Geometry check sheet. Reference: the model listing, model coordinates, mm. A direction names the side the tool comes from. Coordinates: 2 decimals unless noted, no trailing zeros. Order: outer loops, then holes, each group sorted by start corner. A loop starts at its lowest first (then second) coordinate and runs counter-clockwise, first axis right, second up. Notation, with made-up numbers: M -38.5,0.5 L 8.5,0.5 A25 cw 8.5,33.5 Z; hole C 38.25,30 d5. An arc over 180 degrees is marked long. One line per item, written item: value. Start each with the question number.
1) Go/stop test with flat-tipped pins: P1, Ø1.9, axis at x = -44.5, z = -0.5, coming from the -Y side; P2, Ø7, axis at x = -55, z = -5, coming from the -Y side; P3, Ø1.9, axis at y = 14.5, z = -0.5, coming from the -X side. Record where each tip stops, or that it passes through.
2) Access from +Z, -Z, +X, -X, +Y, -Y to the whole of each face (thin tool, end or side, straight path). Record for faces 1 (the flat face through (-54, 25.4, 0)), 2 (the flat face through (-31, 37, -3.175)), 3 (the flat face through (-38, 50.8, 9)).
3) Sectioned sample at A-A, the plane z = -11. Enter the section's corners in (x, y), then the cut area to 3 significant figures.
4) Thickness scan on L1, parallel to X at y = 25, z = 0; L2, parallel to Y at x = -25, z = -1; L3, parallel to Z at x = -9.5, y = 49.5 (3 decimals). Record the ranges inside material, lowest first. Write a range as from..to.
5) Sectioned sample at C-C, the plane y = 3. Enter the section's corners in (x, z) (3 decimals), then the cut area to 3 significant figures.
6) Sectioned sample at D-D, the plane z = -1. Enter the section's corners in (x, y), then the cut area to 3 significant figures.
7) Sectioned sample at B-B, the plane x = -34. Enter the section's corners in (y, z) (3 decimals), then the cut area to 3 significant figures.
```python
from build123d import *

# Parameters (mm, degrees)
F0_W          = 50.8
F0_H          = 50.8
F3_DEPTH      = 3.175
F4_DEPTH      = 15.875
F5_DEPTH      = 15.875
F6_T1_DEPTH   = 28.6978363942
F6_T3_DEPTH   = 28.6978363942
F6_T5_DEPTH   = 28.6978363942
F6_T7_DEPTH   = 28.6978363942
F6_T13_DEPTH  = 31.9956727883
F6_T17_DEPTH  = 31.9956727883
F6_T24_DEPTH  = 31.9956727883
F6_T28_DEPTH  = 31.9956727883
F6_T35_DEPTH  = 31.9956727883
F6_T39_DEPTH  = 31.9956727883
F6_T46_DEPTH  = 31.9956727883
F6_T50_DEPTH  = 31.9956727883
F7_R          = 12.7
F8_DEPTH      = 15.876
F8_DEPTH_BACK = 15.876


# Not quite as in the source:
# - a fillet or chamfer that OpenCascade refuses, or shapes differently, is made with other operations: its cross-section is extruded or revolved along the edge and cut away or added


with BuildPart() as f3:
    # F0 (on Top) → F3 (new body, symmetric)
    with BuildSketch(Plane.XY):
        with Locations((-25.4, 25.4)):
            Rectangle(F0_W, F0_H)
    extrude(amount=F3_DEPTH, both=True)

    # F1 (on Top) → F4 (join, symmetric)
    with BuildSketch(Plane.XY):
        Polygon((0, 25.4), (0, 0), (-25.4, 0), (-25.4, -6.8448194891), (6.35, -6.8448194891), (6.35, 25.4), align=None)
    extrude(amount=F4_DEPTH, both=True)

    # F2 (on Top) → F5 (join, symmetric)
    with BuildSketch(Plane.XY):
        Polygon((-50.8, 50.8), (-25.4, 50.8), (-25.4, 57.15), (-57.15, 57.15), (-57.15, 25.4), (-50.8, 25.4), align=None)
    extrude(amount=F5_DEPTH, both=True)

    # F6: chamfer of 1.27 x 0.3402954744 on 8 edges, made by hand

    # F6_s2 → F6_t1 (cut)
    with BuildSketch(Plane.YZ.offset(-28.6978363942)):
        Polygon((0, 14.605), (-0.3402954744, 15.875), (0, 15.875), align=None)
        Polygon((-1.27, -15.875), (0, -15.5347045256), (0, -15.875), align=None)
    extrude(amount=F6_T1_DEPTH, mode=Mode.SUBTRACT)

    # F6_s4 → F6_t3 (cut)
    with BuildSketch(Plane.XZ.offset(-28.6978363942)):
        Polygon((0, 14.605), (0.3402954744, 15.875), (0, 15.875), align=None)
        Polygon((1.27, -15.875), (0, -15.5347045256), (0, -15.875), align=None)
    extrude(amount=F6_T3_DEPTH, mode=Mode.SUBTRACT)

    # F6_s6 → F6_t5 (cut)
    with BuildSketch(Plane.YZ.offset(-50.8)):
        Polygon((50.8, 14.605), (51.1402954744, 15.875), (50.8, 15.875), align=None)
        Polygon((50.8, -15.5347045256), (52.07, -15.875), (50.8, -15.875), align=None)
    extrude(amount=F6_T5_DEPTH, mode=Mode.SUBTRACT)

    # F6_s8 → F6_t7 (cut)
    with BuildSketch(Plane.XZ.offset(-50.8)):
        Polygon((-50.8, 15.5347045256), (-52.07, 15.875), (-50.8, 15.875), align=None)
        Polygon((-50.8, -14.605), (-51.1402954744, -15.875), (-50.8, -15.875), align=None)
    extrude(amount=F6_T7_DEPTH, mode=Mode.SUBTRACT)


with BuildPart() as f6_tool11:
    # F6_s12 → F6_t13 (new body)
    with BuildSketch(Plane.YZ.offset(3.2978363942)):
        Polygon((0, 14.605), (-0.3402954744, 15.875), (0, 15.875), align=None)
    extrude(amount=-F6_T13_DEPTH)

    split(bisect_by=Plane.YZ, keep=Keep.TOP)


with BuildPart() as f6_tool15:
    # F6_s16 → F6_t17 (new body)
    with BuildSketch(Plane.XZ.offset(-28.6978363942)):
        Polygon((0, 14.605), (0.3402954744, 15.875), (0, 15.875), align=None)
    extrude(amount=F6_T17_DEPTH)

    split(bisect_by=Plane.XZ, keep=Keep.TOP)


with BuildPart() as f6_tool11_1:
    add(f6_tool11.part)

    # F6_t19: intersect F6_tool15
    add(f6_tool15.part, mode=Mode.INTERSECT)


with BuildPart() as f3_1:
    add(f3.part)

    # F6_t9: cut F6_tool11
    add(f6_tool11_1.part, mode=Mode.SUBTRACT)


with BuildPart() as f6_tool22:
    # F6_s23 → F6_t24 (new body)
    with BuildSketch(Plane.YZ.offset(-54.0978363942)):
        Polygon((50.8, 14.605), (51.1402954744, 15.875), (50.8, 15.875), align=None)
    extrude(amount=F6_T24_DEPTH)

    split(bisect_by=Plane.YZ.offset(-50.8), keep=Keep.BOTTOM)


with BuildPart() as f6_tool26:
    # F6_s27 → F6_t28 (new body)
    with BuildSketch(Plane.XZ.offset(-22.1021636058)):
        Polygon((-50.8, 15.5347045256), (-52.07, 15.875), (-50.8, 15.875), align=None)
    extrude(amount=-F6_T28_DEPTH)

    split(bisect_by=Plane.XZ.offset(-50.8), keep=Keep.BOTTOM)


with BuildPart() as f6_tool22_1:
    add(f6_tool22.part)

    # F6_t30: intersect F6_tool26
    add(f6_tool26.part, mode=Mode.INTERSECT)


with BuildPart() as f3_2:
    add(f3_1.part)

    # F6_t20: cut F6_tool22
    add(f6_tool22_1.part, mode=Mode.SUBTRACT)


with BuildPart() as f6_tool33:
    # F6_s34 → F6_t35 (new body)
    with BuildSketch(Plane.XZ.offset(-28.6978363942)):
        Polygon((1.27, -15.875), (0, -15.5347045256), (0, -15.875), align=None)
    extrude(amount=F6_T35_DEPTH)

    split(bisect_by=Plane.XZ, keep=Keep.TOP)


with BuildPart() as f6_tool37:
    # F6_s38 → F6_t39 (new body)
    with BuildSketch(Plane.YZ.offset(3.2978363942)):
        Polygon((-1.27, -15.875), (0, -15.5347045256), (0, -15.875), align=None)
    extrude(amount=-F6_T39_DEPTH)

    split(bisect_by=Plane.YZ, keep=Keep.TOP)


with BuildPart() as f6_tool33_1:
    add(f6_tool33.part)

    # F6_t41: intersect F6_tool37
    add(f6_tool37.part, mode=Mode.INTERSECT)


with BuildPart() as f3_3:
    add(f3_2.part)

    # F6_t31: cut F6_tool33
    add(f6_tool33_1.part, mode=Mode.SUBTRACT)


with BuildPart() as f6_tool44:
    # F6_s45 → F6_t46 (new body)
    with BuildSketch(Plane.YZ.offset(-54.0978363942)):
        Polygon((50.8, -15.5347045256), (52.07, -15.875), (50.8, -15.875), align=None)
    extrude(amount=F6_T46_DEPTH)

    split(bisect_by=Plane.YZ.offset(-50.8), keep=Keep.BOTTOM)


with BuildPart() as f6_tool48:
    # F6_s49 → F6_t50 (new body)
    with BuildSketch(Plane.XZ.offset(-22.1021636058)):
        Polygon((-50.8, -14.605), (-51.1402954744, -15.875), (-50.8, -15.875), align=None)
    extrude(amount=-F6_T50_DEPTH)

    split(bisect_by=Plane.XZ.offset(-50.8), keep=Keep.BOTTOM)


with BuildPart() as f6_tool44_1:
    add(f6_tool44.part)

    # F6_t52: intersect F6_tool48
    add(f6_tool48.part, mode=Mode.INTERSECT)


with BuildPart() as f3_4:
    add(f3_3.part)

    # F6_t42: cut F6_tool44
    add(f6_tool44_1.part, mode=Mode.SUBTRACT)

    # F7 (on Top) → F8 (cut, two sides)
    with BuildSketch(Plane.XY) as f8_sk:
        with Locations((-25.4, 25.4)):
            Circle(F7_R)
    extrude(amount=-F8_DEPTH, mode=Mode.SUBTRACT)
    extrude(f8_sk.sketch, amount=F8_DEPTH_BACK, mode=Mode.SUBTRACT)


solid = f3_4.part
```
Final values:
1. P1: stops at y = 0
1. P2: stops at y = 25.4
1. P3: stops at x = -50.8
2. face 1: +Z, -Z, -X, -Y
2. face 2: -Z
2. face 3: +Z, +X, -Y
3. outline: M -57.15,25.4 L -50.8,25.4 L -50.8,50.8 L -25.4,50.8 L -25.4,57.15 L -57.15,57.15 Z; M -25.4,-6.84 L 6.35,-6.84 L 6.35,25.4 L 0,25.4 L 0,0 L -25.4,0 Z
3. area: 742 mm^2
4. L1: x = -50.8..-38.09, -12.71..6.35
4. L2: y = -6.84..12.71, 38.09..50.8
4. L3: z = -3.175..3.175
5. outline: M -50.8,-3.175 L 0,-3.175 L 0,-15.535 L 1.27,-15.875 L 6.35,-15.875 L 6.35,15.875 L 0.34,15.875 L 0,14.605 L 0,3.175 L -50.8,3.175 Z
5. area: 524 mm^2
6. outline: M -57.15,25.4 L -50.8,25.4 L -50.8,0 L -25.4,0 L -25.4,-6.84 L 6.35,-6.84 L 6.35,25.4 L 0,25.4 L 0,50.8 L -25.4,50.8 L -25.4,57.15 L -57.15,57.15 Z; hole C -25.4,25.4 d25.4
6. area: 2,820 mm^2
7. outline: M 0,-3.175 L 16.055,-3.175 L 16.055,3.175 L 0,3.175 Z; M 34.745,-3.175 L 50.8,-3.175 L 50.8,-15.535 L 52.07,-15.875 L 57.15,-15.875 L 57.15,15.875 L 51.14,15.875 L 50.8,14.605 L 50.8,3.175 L 34.745,3.175 Z
7. area: 405 mm^2
